```python
from build123d import *

# Parameters (mm, degrees)
SKETCH_W        = 150
SKETCH_H        = 150
PAD_DEPTH       = 5
SKETCH001_R     = 1.5
POCKET_DEPTH    = 6
POCKET001_DEPTH = 6
SKETCH003_R     = 1.5
POCKET002_DEPTH = 6
SKETCH004_R     = 2.5
POCKET003_DEPTH = 2


with BuildPart() as part:
    # Sketch → Pad (new body)
    with BuildSketch(Plane.XY):
        Rectangle(SKETCH_W, SKETCH_H)
    extrude(amount=PAD_DEPTH)

    # Sketch001 (on Face6 of Pad) → Pocket (cut)
    with BuildSketch(Plane.XY.offset(5)):
        with Locations((-63.698635, 62.476162)):
            Circle(SKETCH001_R)
        with Locations((55.516754, 61.662395)):
            Circle(SKETCH001_R)
        with Locations((62.026806, -67.318062)):
            Circle(SKETCH001_R)
        with Locations((-64.51239, -66.911179)):
            Circle(SKETCH001_R)
        with Locations((-15.987179, 0)):
            Circle(SKETCH001_R)
        with Locations((15.989725, 0)):
            Circle(SKETCH001_R)
        Polygon((-78.334322, 45.976028), (-43.69331, 25.97602), (-43.69331, -26.515585), (-78.334322, -46.515593), align=None)
        Polygon((76.538069, 49.887789), (41.89705, 29.887793), (41.89705, -27.543442), (76.538069, -47.543438), align=None)
    extrude(amount=-POCKET_DEPTH, mode=Mode.SUBTRACT)

    # Sketch002 (on Face5 of Pocket) → Pocket001 (cut)
    with BuildSketch(Plane.XY.offset(5)):
        with BuildLine():
            ThreePointArc((-76.389725, -59.129343), (-71.755036, -69.691564), (-62.212372, -76.170639))
            Line((-62.212372, -76.170639), (-76.389725, -76.170639))
            Line((-76.389725, -59.129343), (-76.389725, -76.170639))
        make_face()
        with BuildLine():
            ThreePointArc((76.179779, 60.880058), (70.14646, 71.330769), (59.165479, 76.334403))
            Line((59.165479, 76.334403), (75.819939, 75.661225))
            Line((76.179779, 60.880058), (75.819939, 75.661225))
        make_face()
        with BuildLine():
            ThreePointArc((60.306034, -75.499916), (70.844496, -69.462138), (75.808842, -58.377499))
            Line((75.808842, -58.377499), (75.280468, -75.273705))
            Line((60.306034, -75.499916), (75.280468, -75.273705))
        make_face()
        with BuildLine():
            ThreePointArc((-57.073154, 76.163305), (-69.273576, 71.27005), (-75.626793, 59.762188))
            Line((-75.626793, 59.762188), (-75.289242, 75.58445))
            Line((-57.073154, 76.163305), (-75.289242, 75.58445))
        make_face()
    extrude(amount=-POCKET001_DEPTH, mode=Mode.SUBTRACT)

    # Sketch003 (on Face4 of Pocket001) → Pocket002 (cut)
    with BuildSketch(Plane.XY.offset(5)):
        with Locations((-19.585, 60.455048)):
            Circle(SKETCH003_R)
        with Locations((19.585, 60.455048)):
            Circle(SKETCH003_R)
        with Locations((19.585, -60.455048)):
            Circle(SKETCH003_R)
        with Locations((-19.585, -60.455048)):
            Circle(SKETCH003_R)
    extrude(amount=-POCKET002_DEPTH, mode=Mode.SUBTRACT)

    # Sketch004 (on Face4 of Pocket002) → Pocket003 (cut)
    with BuildSketch(Plane.XY.offset(5)):
        with Locations((-15.954409, 0)):
            Circle(SKETCH004_R)
        with Locations((15.993672, 0)):
            Circle(SKETCH004_R)
    extrude(amount=-POCKET003_DEPTH, mode=Mode.SUBTRACT)


solid = part.part
```
CAD build for the part. Positions are in the model's coordinates, mm. A direction names the side the tool comes from. Coordinates: 2 decimals unless noted, no trailing zeros. Order: outer loops, then holes, each group sorted by start corner. A loop starts at its lowest first (then second) coordinate and runs counter-clockwise, first axis right, second up. Notation, with made-up numbers: (57, 21) - (103, 21) arc R11 cw to (103, 26) - close; hole circle Ø6 at (50.5, 18). An arc over 180 degrees is marked (long way). Answer in a Markdown table with one row per item.
1. Slice it at B-B, the plane y = 19.5. List the corners of the cut face in (x, z).
Answer:
| item | result |
|---|---|
| outline | (-43.69, 0) - (41.9, 0) - (41.9, 5) - (-43.69, 5) - close |
2. Flat gauge pins, fed straight in: P1, Ø1.5, axis at y = -2.5, z = 1.5, coming from the +X side; P2, Ø2.5, axis at x = 16.5, y = -0.5, coming from the +Z side; P3, Ø2, axis at y = 38.5, z = 0.5, coming from the +X side. Where does each tip first touch, or does it go through?
Answer:
| item | result |
|---|---|
| P1 | x = 41.9 |
| P2 | z = 3 |
| P3 | x = 58.55 |
3. Slice it at C-C, the plane y = -41.5. List the corners of the cut face in (x, z).
Answer:
| item | result |
|---|---|
| outline | (-69.65, 0) - (66.07, 0) - (66.07, 5) - (-69.65, 5) - close |
4. Slice it at A-A, the plane z = 2.15. Give the number of separate pieces and of enclosed holes in the cut face, then the cut area to 3 significant figures.
Answer:
| item | result |
|---|---|
| separate pieces | 1 |
| enclosed holes | 10 |
| area | 17,500 mm² |
5. 3-axis set-ups, long thin cutter, end or side, ignore diameter. For faces 1 (the face through (18.38, 0.75, 4.01)), 2 (the face through (58.217, -36.966, 2.535)), 3 (the face through (-59.566, 35.14, 2.535)): which of +Z, -Z, +X, -X, +Y, -Y reach the whole face in a straight line?
Answer:
| item | result |
|---|---|
| face 1 | +Z |
| face 2 | +Z, -Z, +X |
| face 3 | +Z, -Z, -X |
6. Pull direction X, two halves, no side cores. Call faces 4 (the face through (0, 75, 2)), 5 (the face through (-71.068, -70.477, 2.535)), 6 (the face through (18, 0, 3)), 7 (the face through (-13.57, 0.75, 4.01)): +X half, -X half, draft (parallel to the pull), parting line (faces both ways), or undercut.
Answer:
| item | result |
|---|---|
| face 4 | draft |
| face 5 | -X half |
| face 6 | undercut |
| face 7 | undercut |
7. Drill centre lines: L1, parallel to Y at x = -16, z = 4.15; L2, parallel to Y at x = 19, z = 2.95; L3, parallel to X at y = -14, z = 4.7. Where is each one in solid material? Low to high. Write a range as from..to.
Answer:
| item | result |
|---|---|
| L1 | -75..-2.5, 2.5..75 |
| L2 | -75..-61.84, -59.07..59.07, 61.84..75 |
| L3 | -43.69..41.9 |
